Verification items for the finished model (mm, model axes). Face numbers are marked on the shaded views. A direction names the side the tool comes from. Give positions to 0.01 mm unless a question says otherwise; leave off trailing zeros. Loops run counter-clockwise (first coordinate to the right, second up) from the corner with the lowest first, then second, coordinate; pieces in that order, holes last. Notation, with made-up numbers: M 21.25,70 L 68.25,70 A26 cw 68.25,94 Z; hole C 73.25,88.5 d2. An arc over 180 degrees is marked long. Use a Markdown table: item, result.
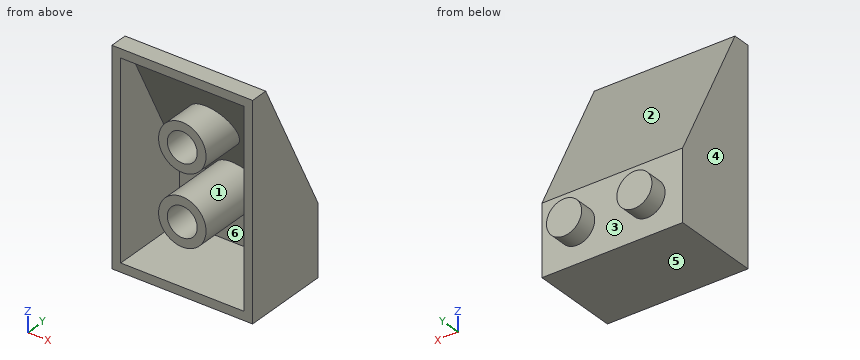
from build123d import *

# Parameters (mm, degrees)
BOSS_EXTRUDE1_DEPTH = 16
SKETCH2_R           = 2
BOSS_EXTRUDE2_DEPTH = 2
SHELL1_T            = -1
BOSS_EXTRUDE3_REACH = 14
SKETCH3_R           = 2.7
SKETCH3_R_2         = 1.7


with BuildPart() as part:
    # Sketch1 → Boss-Extrude1 (new body)
    with BuildSketch(Plane(origin=(0, 0, 0), x_dir=(0, 0, -1), z_dir=(1, 0, 0))):
        Polygon((0, 0), (0, 10), (-8, 10), (-24, 2), (-24, 0), align=None)
    extrude(amount=BOSS_EXTRUDE1_DEPTH)

    # Sketch2 → Boss-Extrude2 (add)
    with BuildSketch(Plane(origin=(0, 10, 0), x_dir=(1, 0, 0), z_dir=(0, 1, 0))):
        with Locations((4, -4)):
            Circle(SKETCH2_R)
        with Locations((12, -4)):
            Circle(SKETCH2_R)
    extrude(amount=BOSS_EXTRUDE2_DEPTH)

    # Shell1
    shell1_openings = [part.faces().sort_by_distance(p)[0] for p in [
        (8, 0, 12),
    ]]
    offset(amount=SHELL1_T, openings=shell1_openings, kind=Kind.INTERSECTION)

    # Sketch3 → Boss-Extrude3 (add, up to next)
    with BuildSketch(Plane.XZ, mode=Mode.PRIVATE) as boss_extrude3_sk1:
        with Locations((8, 8)):
            Circle(SKETCH3_R)
        with Locations((8, 8)):
            Circle(SKETCH3_R_2, mode=Mode.SUBTRACT)
    boss_extrude3_tool1 = extrude(boss_extrude3_sk1.sketch, amount=-BOSS_EXTRUDE3_REACH, mode=Mode.PRIVATE) - part.part
    add(boss_extrude3_tool1.solids().sort_by_distance((5.376368, 0, 8))[0])
    # Sketch3 → Boss-Extrude3 (add, up to next)
    with BuildSketch(Plane.XZ, mode=Mode.PRIVATE) as boss_extrude3_sk2:
        with Locations((8, 16)):
            Circle(SKETCH3_R)
        with Locations((8, 16)):
            Circle(SKETCH3_R_2, mode=Mode.SUBTRACT)
    boss_extrude3_tool2 = extrude(boss_extrude3_sk2.sketch, amount=-BOSS_EXTRUDE3_REACH, mode=Mode.PRIVATE) - part.part
    add(boss_extrude3_tool2.solids().sort_by_distance((5.376368, 0, 16))[0])


solid = part.part
(1) Draft check along Z on the marked faces 4, 5 and 6. Enter one of: +Z half, -Z half, draft (parallel to the pull), parting line (faces both ways), or undercut.
Results below:
| item | result |
|---|---|
| face 4 | draft |
| face 5 | -Z half |
| face 6 | undercut |
(2) Cross-section at A-A on y = 0.75. Record the cut outline in (x, z), then the cut area to 3 significant figures.
Results below:
| item | result |
|---|---|
| outline | M 0,0 L 16,0 L 16,24 L 0,24 Z; C 8,8 d5.4; C 8,16 d5.4; hole M 1,1 L 15,1 L 15,23 L 1,23 Z; hole C 8,8 d3.4; hole C 8,16 d3.4 |
| area | 104 mm^2 |
(3) Cross-section at D-D on z = 6.75. Record the cut outline in (x, y), then the cut area to 3 significant figures.
Results below:
| item | result |
|---|---|
| outline | M 0,0 L 1,0 L 1,9 L 5.61,9 L 5.61,0 L 6.85,0 L 6.85,9 L 9.15,9 L 9.15,0 L 10.39,0 L 10.39,9 L 15,9 L 15,0 L 16,0 L 16,10 L 0,10 Z |
| area | 56.3 mm^2 |
(4) Set-up check for the marked faces 1, 2 and 3: record each of +Z, -Z, +X, -X, +Y, -Y from which the full face is reachable in a straight line by a thin tool's end or side.
Results below:
| item | result |
|---|---|
| face 1 | -Y |
| face 2 | +Z, +X, -X, +Y |
| face 3 | +Y |
(5) Material ranges on line 1 (X direction, y = 6.75, z = 8); line 2 (Z direction, x = 4, y = 10.45); line 3 (X direction, y = 4.5, z = 9), recorded low to high.
Results below:
| item | result |
|---|---|
| line 1 | 0 to 1, 5.3 to 6.3, 9.7 to 10.7, 15 to 16 |
| line 2 | 2 to 3, 5 to 6 |
| line 3 | 0 to 1, 5.49 to 6.63, 9.37 to 10.51, 15 to 16 |
(6) Cross-section at B-B on x = 1.25. Record the cut outline in (y, z), then the cut area to 3 significant figures.
Results below:
| item | result |
|---|---|
| outline | M 0,0 L 10,0 L 10,8 L 2,24 L 0,24 L 0,23 L 1.38,23 L 9,7.76 L 9,1 L 0,1 Z |
| area | 36.0 mm^2 |
(7) Cross-section at C-C on y = 7. Record the cut outline in (x, z).
Results below:
| item | result |
|---|---|
| outline | M 0,0 L 16,0 L 16,14 L 0,14 Z; C 8,8 d5.4; hole M 1,1 L 15,1 L 15,11.76 L 1,11.76 Z; hole C 8,8 d3.4 |
(8) Gauge pin test, flat ends, axial feed: P1, Ø4.5, axis at y = 2.5, z = 10, coming from the -X side; P2, Ø0.6, axis at x = 11.5, z = 4, coming from the -Y side; P3, Ø4, axis at x = 8, z = 16, coming from the +Y side; P4, Ø1.5, axis at y = 6.5, z = 20.5, coming from the +X side. Record the tip position at first contact, or that the pin passes through.
Results below:
| item | result |
|---|---|
| P1 | x = 0 |
| P2 | y = 11 |
| P3 | y = 7 |
| P4 | through |
